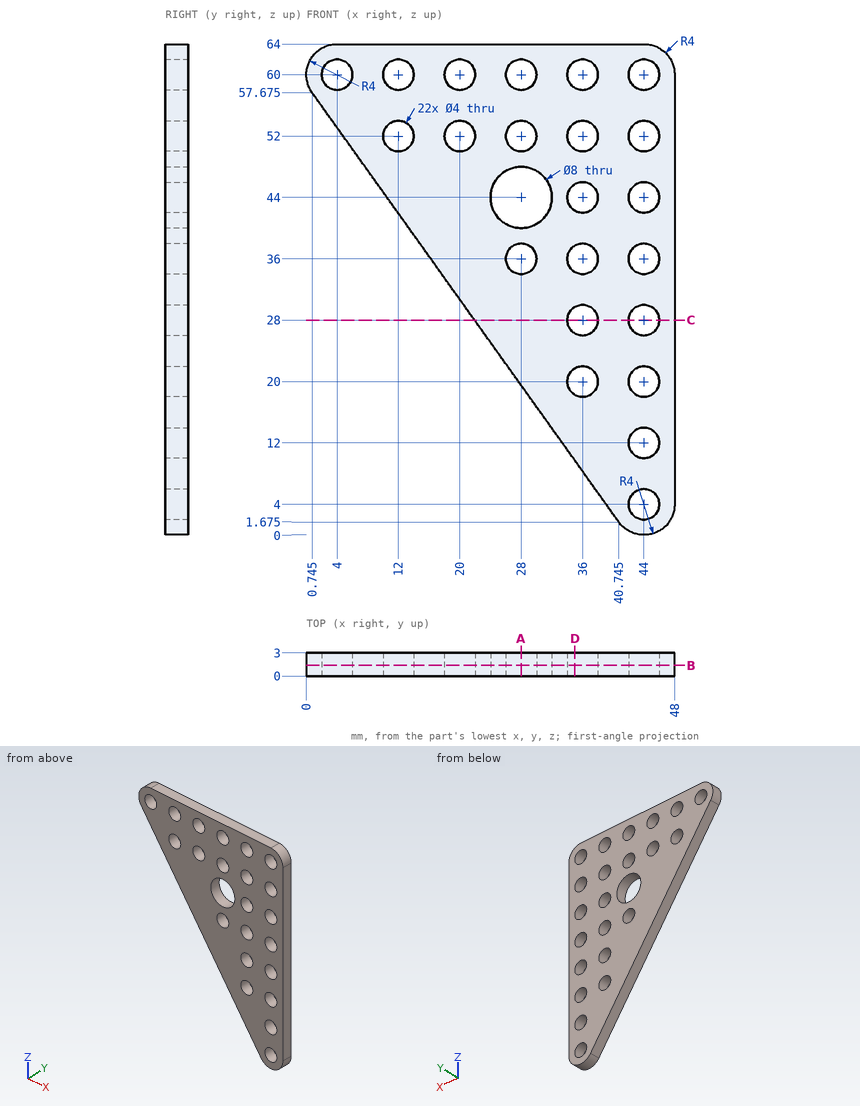
Design review of the part shown in the three views and the two pictorial views. Dimensions are in mm from the part's minimum x, y and z. Round coordinates to 2 decimals unless told otherwise and drop trailing zeros. Loops run counter-clockwise (first coordinate to the right, second up) from the corner with the lowest first, then second, coordinate; pieces in that order, holes last. Notation, with made-up numbers: (-19, -27.5) -> (6, -27.5) arc R36 ccw to (6, 8.5) -> close; hole circle Ø2 at (81, -35). An arc over 180 degrees is marked (long way). Answer as CSV lines item,"result".
1) Add section C-C on z = 28. Write out the cut boundary in (x, y).
Geometry results:
outline,"(21.94, 0) -> (34, 0) -> (34, 3) -> (21.94, 3) -> close; (38, 0) -> (42, 0) -> (42, 3) -> (38, 3) -> close; (46, 0) -> (48, 0) -> (48, 3) -> (46, 3) -> close"
2) Add section B-B on y = 1.4. State how many separate pieces and enclosed holes the cut face has, plus the area to 3 significant figures.
Geometry results:
separate pieces,"1"
enclosed holes,"23"
area,"1,500 mm²"
3) To check wall thickness, follow line 1 along X through (y, z) = (2.5, 20); line 2 along X through (y, z) = (1.9, 44); line 3 along X through (y, z) = (0.8, 28). State the ranges of each line that lie inside material, in increasing order. Write a range as from..to.
Geometry results:
line 1,"x = 27.66..34, 38..42, 46..48"
line 2,"x = 10.51..24, 32..34, 38..42, 46..48"
line 3,"x = 21.94..34, 38..42, 46..48"
4) Add section A-A on x = 28. Write out the cut boundary in (y, z).
Geometry results:
outline,"(0, 19.52) -> (3, 19.52) -> (3, 34) -> (0, 34) -> close; (0, 38) -> (3, 38) -> (3, 40) -> (0, 40) -> close; (0, 48) -> (3, 48) -> (3, 50) -> (0, 50) -> close; (0, 54) -> (3, 54) -> (3, 58) -> (0, 58) -> close; (0, 62) -> (3, 62) -> (3, 64) -> (0, 64) -> close"
5) Add section D-D on x = 35. Write out the cut boundary in (y, z).
Geometry results:
outline,"(0, 9.72) -> (3, 9.72) -> (3, 18.27) -> (0, 18.27) -> close; (0, 21.73) -> (3, 21.73) -> (3, 26.27) -> (0, 26.27) -> close; (0, 29.73) -> (3, 29.73) -> (3, 34.27) -> (0, 34.27) -> close; (0, 37.73) -> (3, 37.73) -> (3, 42.27) -> (0, 42.27) -> close; (0, 45.73) -> (3, 45.73) -> (3, 50.27) -> (0, 50.27) -> close; (0, 53.73) -> (3, 53.73) -> (3, 58.27) -> (0, 58.27) -> close; (0, 61.73) -> (3, 61.73) -> (3, 64) -> (0, 64) -> close"
6) For P1, Ø3.5, axis at x = 12, z = 52, coming from the +Y side, flat-tipped, find the tip position at first contact; note if it passes through.
Geometry results:
P1,"passes through"
